```python
from build123d import *

# Parameters (mm, degrees)
SKETCH1_W           = 228.6
SKETCH1_H           = 304.8
BOSS_EXTRUDE1_DEPTH = 12.7
CUT_EXTRUDE1_DEPTH  = 9.525
CHAMFER1_SIZE       = 4.7625
CHAMFER2_SIZE       = 3.175


with BuildPart() as part:
    # Sketch1 → Boss-Extrude1 (new body)
    with BuildSketch(Plane.XY):
        Rectangle(SKETCH1_W, SKETCH1_H)
    extrude(amount=BOSS_EXTRUDE1_DEPTH)

    # Sketch2 → Cut-Extrude1 (cut)
    with BuildSketch(Plane.XY.offset(12.7)):
        with BuildLine():
            Line((97.95, -142.4), (-97.95, -142.4))
            ThreePointArc((-97.95, -142.4), (-102.440128061, -140.540128061), (-104.3, -136.05))
            Line((-104.3, -136.05), (-104.3, 136.05))
            ThreePointArc((-104.3, 136.05), (-102.440128061, 140.540128061), (-97.95, 142.4))
            Line((-97.95, 142.4), (97.95, 142.4))
            ThreePointArc((97.95, 142.4), (102.440128061, 140.540128061), (104.3, 136.05))
            Line((104.3, 136.05), (104.3, -136.05))
            ThreePointArc((104.3, -136.05), (102.440128061, -140.540128061), (97.95, -142.4))
        make_face()
    extrude(amount=-CUT_EXTRUDE1_DEPTH, mode=Mode.SUBTRACT)

    # Chamfer1
    chamfer1_edges = [part.edges().sort_by_distance(p)[0] for p in [
        (-114.3, 152.4, 6.35),
        (114.3, 152.4, 6.35),
        (114.3, -152.4, 6.35),
        (-114.3, -152.4, 6.35),
    ]]
    chamfer(chamfer1_edges, length=CHAMFER1_SIZE)

    # Chamfer2
    chamfer2_edges = [part.edges().sort_by_distance(p)[0] for p in [
        (0, -152.4, 12.7),
        (-114.3, 0, 12.7),
        (114.3, 0, 12.7),
        (0, 152.4, 12.7),
        (111.91875, 150.01875, 12.7),
        (-111.91875, 150.01875, 12.7),
        (111.91875, -150.01875, 12.7),
        (-111.91875, -150.01875, 12.7),
    ]]
    chamfer(chamfer2_edges, length=CHAMFER2_SIZE)


solid = part.part
```
Geometry: final body of the model. Coordinates: model frame, mm. A direction names the side the tool comes from. Coordinates: 2 decimals unless noted, no trailing zeros. Order: outer loops, then holes, each group sorted by start corner. A loop starts at its lowest first (then second) coordinate and runs counter-clockwise, first axis right, second up. Notation, with made-up numbers: (-2.5, -30) - (41.5, -30) arc R20 ccw to (41.5, -21) - close; hole circle Ø7 at (68.25, 56.25). An arc over 180 degrees is marked (long way). Return JSON: item names as keys, results as strings. Group by question number.
1. Cut plane B-B (x = 57). Output: boundary loops of the cut face in (y, z) (3 decimals).
2. Pin query (flat end, axial travel): pin 1 (3 mm diameter, centred on x = 9, y = -83, fed in from +Z) (3 decimals). Return the tip coordinate at first contact, or that it passes through.
3. Material intervals for line 1 along X through (y, z) = (-94, 6.75); line 2 along Y through (x, z) = (-24, 4.75); line 3 along Z through (x, y) = (28, 101) (3 decimals), sorted ascending. Write a range as [from, to].
4. Cut plane A-A (y = -75). Output: boundary loops of the cut face in (x, z) (3 decimals).
5. Set-up query: faces 1 (the face through (-110.814, 148.847, 11.135)), 2 (the face through (-1, 142.4, 8)). Return all of +Z, -Z, +X, -X, +Y, -Y with unobstructed straight access to the full face (end or side cutting, diameter ignored); none if empty.
6. Pull-direction query (X, two-part tool) for faces 3 (the face through (110.779, -148.945, 11.09)), 4 (the face through (-102.39, -140.59, 8)), 5 (the face through (102.49, -140.49, 8)), 6 (the face through (-108, 1, 12.7)); classes: pulls with the +X half, pulls with the -X half, needs draft (parallel to the pull), parting line crosses it, or undercut.
Resolved:
{
 "1": {"outline": "(-152.4, 0) - (152.4, 0) - (152.4, 9.525) - (149.225, 12.7) - (142.4, 12.7) - (142.4, 3.175) - (-142.4, 3.175) - (-142.4, 12.7) - (-149.225, 12.7) - (-152.4, 9.525) - close"},
 "2": {"pin 1": "stops at z = 3.175"},
 "3": {"line 1": "x = [-114.3, -104.3], [104.3, 114.3]", "line 2": "y = [-152.4, -142.4], [142.4, 152.4]", "line 3": "z = [0, 3.175]"},
 "4": {"outline": "(-114.3, 0) - (114.3, 0) - (114.3, 9.525) - (111.125, 12.7) - (104.3, 12.7) - (104.3, 3.175) - (-104.3, 3.175) - (-104.3, 12.7) - (-111.125, 12.7) - (-114.3, 9.525) - close"},
 "5": {"face 1": "+Z, -X, +Y", "face 2": "+Z"},
 "6": {"face 3": "pulls with the +X half", "face 4": "undercut", "face 5": "undercut", "face 6": "needs draft"}
}
